Geometry: see drawing. Coordinates: mm, zero at the bounding-box minimum. Give positions to 0.01 mm unless a question says otherwise; leave off trailing zeros. Loops run counter-clockwise (first coordinate to the right, second up) from the corner with the lowest first, then second, coordinate; pieces in that order, holes last. Notation, with made-up numbers: M -35,29 L -26,29 A12 cw -26,48 Z; hole C 12.5,32.25 d2. An arc over 180 degrees is marked long. Put each result on its own line as item: value.
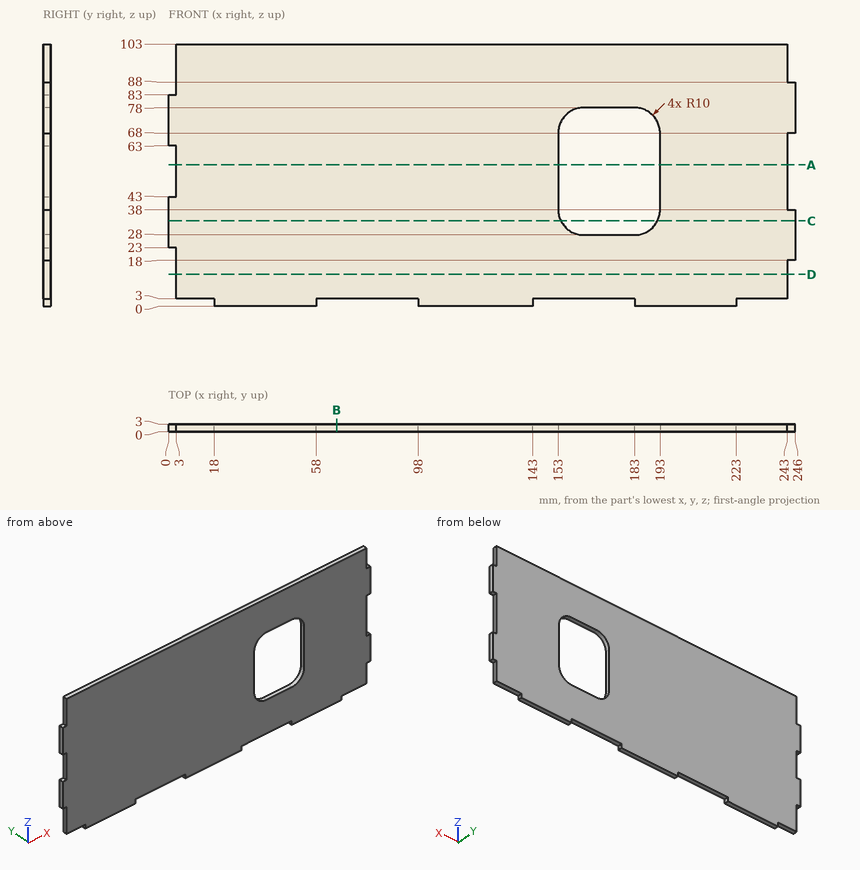
Item 1: Section C-C on z = 33.5. Output: boundary loops of the cut face in (x, y), then the cut area to 3 significant figures.
Output values:
outline: M 0,0 L 154.07,0 L 154.07,3 L 0,3 Z; M 191.93,0 L 246,0 L 246,3 L 191.93,3 Z
area: 624 mm²
Item 2: Pin query (flat end, axial travel): pin 1 Ø1.5 at (y, z) = (1.5, 1.5) entering from +X; pin 2 Ø1.5 at (y, z) = (2, 59.5) entering from +X; pin 3 Ø0.9 at (x, y) = (1, 1.5) entering from -Z. Return the tip coordinate at first contact, or that it passes through.
Output values:
pin 1: x = 223
pin 2: x = 243
pin 3: z = 23
Item 3: Section A-A on z = 55.5. Output: boundary loops of the cut face in (x, y), then the cut area to 3 significant figures.
Output values:
outline: M 3,0 L 153,0 L 153,3 L 3,3 Z; M 193,0 L 243,0 L 243,3 L 193,3 Z
area: 600 mm²
Item 4: Section B-B on x = 66. Output: boundary loops of the cut face in (y, z), then the cut area to 3 significant figures.
Output values:
outline: M 0,3 L 3,3 L 3,103 L 0,103 Z
area: 300 mm²
Item 5: Section D-D on z = 12.5. Output: boundary loops of the cut face in (x, y).
Output values:
outline: M 3,0 L 243,0 L 243,3 L 3,3 Z
Item 6: Line query: probe 1 along X at (y, z) = (0.45, 64.5); probe 2 along Z at (x, y) = (178.5, 1.05); probe 3 along X at (y, z) = (2.35, 56). Output: solid intervals per line, ascending. Write a range as [from, to].
Output values:
probe 1: [0, 153], [193, 243]
probe 2: [3, 28], [78, 103]
probe 3: [3, 153], [193, 243]
